Autodesk Inventor part; units mm, degrees
ref_plane "YZ Plane" through (0, 0, 0) normal (1, 0, 0) x (0, 1, 0)
ref_plane "XZ Plane" through (0, 0, 0) normal (0, 1, 0) x (-1, 0, 0)
ref_plane "XY Plane" through (0, 0, 0) normal (0, 0, 1) x (1, 0, 0)
sketch "Sketch1" plane through (0, 0, 0) normal (0, 0, 1) x (1, 0, 0)
  circle A0 centre (0, 0) radius 25 construction
  line L0 (0, 0) -> (0, 25) construction
  line L1 (0, 0) -> (21.6506, -12.5) construction
  line L2 (0, 0) -> (-21.6506, -12.5) construction
  line L3 (0, 25) -> (8, 25)
  line L4 (0, 25) -> (-8, 25)
  line L5 (0, 25) -> (8, 25) construction
  line L6 (21.6506, -12.5) -> (25.6506, -5.5718)
  line L7 (21.6506, -12.5) -> (29.6506, -12.5) construction
  line L8 (21.6506, -12.5) -> (17.6506, -19.4282)
  line L9 (21.6506, -12.5) -> (29.6506, -12.5) construction
  line L10 (-21.6506, -12.5) -> (-25.6506, -5.5718)
  line L11 (-21.6506, -12.5) -> (-13.6506, -12.5) construction
  line L12 (-21.6506, -12.5) -> (-17.6506, -19.4282)
  line L13 (-21.6506, -12.5) -> (-13.6506, -12.5) construction
  line L14 (8, 25) -> (8, 34.0735)
  line L15 (-8, 25) -> (-8, 34.0735)
  line L16 (25.6506, -5.5718) -> (33.5085, -10.1085)
  line L17 (17.6506, -19.4282) -> (25.5085, -23.9649)
  line L18 (-17.6506, -19.4282) -> (-25.5085, -23.9649)
  line L19 (-25.6506, -5.5718) -> (-33.5085, -10.1085)
  arc A1 (33.5085, -10.1085) -> (8, 34.0735) centre (0, 0) ccw
  arc A2 (-8, 34.0735) -> (-33.5085, -10.1085) centre (0, 0) ccw
  arc A3 (-25.5085, -23.9649) -> (25.5085, -23.9649) centre (0, 0) ccw
  dimension "d0" = 50
  dimension "d1" = 120
  dimension "d2" = 120
  dimension "d3" = 8
  dimension "d4" = 8
  dimension "d5" = 180
  dimension "d6" = 8
  dimension "d7" = 60
  dimension "d8" = 8
  dimension "d9" = 120
  dimension "d10" = 8
  dimension "d11" = 120
  dimension "d12" = 8
  dimension "d13" = 60
  dimension "d15" = 35
  dimension "d16" = 35
  dimension "d17" = 35
extrude "Extrusion1" add sketch "Sketch1" along normal blind 21
sketch "Sketch2" plane through (0, 0, 21) normal (0, 0, 1) x (1, 0, 0)
  line L0 (-17.5, -17.5) -> (17.5, -17.5)
  line L1 (17.5, -17.5) -> (17.5, 17.5)
  line L2 (17.5, 17.5) -> (-17.5, 17.5)
  line L3 (-17.5, 17.5) -> (-17.5, -17.5)
  line L4 (-17.5, -17.5) -> (17.5, 17.5) construction
  line L5 (17.5, -17.5) -> (-17.5, 17.5) construction
  point P0 (0, 0)
  dimension "d20" = 35
  dimension "d21" = 35
extrude "Extrusion2" add sketch "Sketch2" along normal blind 60
fillet "Fillet1" radius 5 4 edges at (17.5, 17.5, 51) (17.5, -17.5, 51) (-17.5, 17.5, 51) (-17.5, -17.5, 51)
fillet "Fillet2" radius 1 38 edges at (30.3109, 17.5, 0) (-30.3109, 17.5, 0) (0, -35, 0) (21.6506, -12.5, 0) (29.5796, -7.8402, 0) (21.5796, -21.6966, 0) (8, 29.5367, 0) (0, 25, 0) (-8, 29.5367, 0) (-29.5796, -7.8402, 0) (-21.6506, -12.5, 0) (-21.5796, -21.6966, 0) (16.0355, 16.0355, 21) (17.5, 0, 21) (16.0355, -16.0355, 21) (0, -17.5, 21) (-16.0355, -16.0355, 21) (-17.5, 0, 21) (-16.0355, 16.0355, 21) (0, 17.5, 21) (-30.3109, 17.5, 21) (-8, 29.5367, 21) (0, 25, 21) (8, 29.5367, 21) (30.3109, 17.5, 21) (29.5796, -7.8402, 21) (21.6506, -12.5, 21) (21.5796, -21.6966, 21) (0, -35, 21) (-21.5796, -21.6966, 21) (-21.6506, -12.5, 21) (-29.5796, -7.8402, 21) (-8, 34.0735, 10.5) (8, 34.0735, 10.5) (33.5085, -10.1085, 10.5) (25.5085, -23.9649, 10.5) (-25.5085, -23.9649, 10.5) (-25.6506, -5.5718, 10.5)
sketch "Sketch4" plane through (0, 0, 81) normal (0, 0, 1) x (1, 0, 0)
  line L0 (-100, 50) -> (100, 50)
  line L1 (100, 50) -> (100, -50)
  line L2 (100, -50) -> (-100, -50)
  line L3 (-100, -50) -> (-100, 50)
  line L4 (-100, 50) -> (100, -50) construction
  line L5 (100, 50) -> (-100, -50) construction
  point P0 (0, 0)
  dimension "d29" = 200
  dimension "d30" = 100
extrude "Extrusion4" add sketch "Sketch4" along normal blind 39
equation "\"d3\" = d4"
equation "\"d6\" = d4"
equation "\"d8\" = d4"
equation "\"d10\" = d4"
equation "\"d12\" = d4"
equation "\"d16\" = d15"
equation "\"d17\" = d15"
properties part number "Sponge"
Input: part model. Units: mm. Frame: model coordinates. A direction names the side the tool comes from. Give positions to 0.01 mm unless a question says otherwise; leave off trailing zeros. Write each loop counter-clockwise with the first axis right and the second up, starting at its lowest first coordinate (ties: lowest second). Pieces come first, ordered by that corner, then holes. Notation, with made-up numbers: M 57.5,54 L 108.5,54 A26 cw 108.5,78 Z; hole C 38.5,56 d10. An arc over 180 degrees is marked long. Write item = value, one per line. Start each with the question number.
1) Cut plane A-A on z = 37. Return the cut outline in (x, y), then the cut area to 3 significant figures.
2) Cut plane C-C on x = 21. Count the separate pieces of the cut face and the enclosed holes in it, then the cut area to 3 significant figures.
3) First-contact query: pin 1 Ø8 at (y, z) = (3.5, 41) entering from +X; pin 2 Ø7.5 at (x, z) = (0.5, 46.5) entering from +Y; pin 3 Ø4 at (y, z) = (30, 11) entering from -X. Flat tips, straight axial feed; report the tip coordinate or a pass-through.
4) Material intervals for line 1 along Z through (x, y) = (-33, -4); line 2 along Z through (x, y) = (-37, 40); line 3 along Y through (x, z) = (-12.5, 21.5), sorted ascending. Write a range as [from, to].
5) Reachability of faces 1 (the flat face through (-17.5, 0, 51)), 2 (the cylindrical face through (21.33, -12.46, 0.29)), 3 (the cylindrical face through (16, -16.07, 51.91)), 4 (the flat face through (0, 17.5, 51)), 5 (the cylindrical face through (0, -35, 10)) from +Z, -Z, +X, -X, +Y, -Y: full face, straight path, thin tool, end or side. Return the list, or none.
6) Cut plane B-B on x = -62.5. Return the cut outline in (y, z).
7) Draft query along Y for faces 6 (the cylindrical face through (-20.834, -13.313, 20.715)), 7 (the cylindrical face through (30.12, 17.83, 10.37)), 8 (the flat face through (1, -50, 100)). Return one class per face: +Y half, -Y half, draft (parallel to the pull), parting line (faces both ways), or undercut.
Solved:
q1.outline = M -17.5,-12.5 A5 ccw -12.5,-17.5 L 12.5,-17.5 A5 ccw 17.5,-12.5 L 17.5,12.5 A5 ccw 12.5,17.5 L -12.5,17.5 A5 ccw -17.5,12.5 Z
q1.area = 1,200 mm2
q2.separate_pieces = 3
q2.enclosed_holes = 0
q2.area = 4,910 mm2
q3.pin_1 = 17.5
q3.pin_2 = 17.5
q3.pin_3 = -21
q4.line_1 = [0, 21], [81, 120]
q4.line_2 = [81, 120]
q4.line_3 = [-17.63, 17.63]
q5.face_1 = -X, +Y, -Y
q5.face_2 = -Z
q5.face_3 = +X, -Y
q5.face_4 = +X, -X, +Y
q5.face_5 = -Z, -Y
q6.outline = M -50,81 L 50,81 L 50,120 L -50,120 Z
q7.face_6 = undercut
q7.face_7 = parting line
q7.face_8 = -Y half
